```python
from build123d import *


with BuildPart() as part:
    # 스케치2 → 회전1 (revolve)
    with BuildSketch(Plane(origin=(0, 0, 0), x_dir=(0, 0, -1), z_dir=(1, 0, 0))):
        with BuildLine():
            Line((10.1, 0), (12.1, 0))
            ThreePointArc((12.1, 0), (12.521081242, -1.48943877), (11.796548935, -2.857207098))
            ThreePointArc((11.796548935, -2.857207098), (11.081359136, -4.188050052), (11.796542721, -5.518896345))
            ThreePointArc((11.796542721, -5.518896345), (12.753495116, -6.567634704), (13.1, -7.944422413))
            Line((13.1, -7.944422413), (13.1, -19.359260843))
            ThreePointArc((13.1, -19.359260843), (11.975073546, -22.075073546), (9.259260843, -23.2))
            Line((9.259260843, -23.2), (0, -23.2))
            Line((0, -23.2), (0, -20.2))
            Line((0, -20.2), (10.1, -20.2))
            Line((10.1, -20.2), (10.1, 0))
        make_face()
    revolve(axis=Axis((0, -20.2, 0), (0, 1, 0)))


solid = part.part
```
CAD build for the part. Positions are in the model's coordinates, mm. Round coordinates to 2 decimals unless told otherwise and drop trailing zeros. Order: outer loops, then holes, each group sorted by start corner. A loop starts at its lowest first (then second) coordinate and runs counter-clockwise, first axis right, second up. Notation, with made-up numbers: (-1.75, 40.5) -> (19.25, 40.5) arc R21 cw to (19.25, 66.5) -> close; hole circle Ø8 at (49.5, -10.75). An arc over 180 degrees is marked (long way). Write item = value, one per line.
(1) Cut at B-B (z = 0). Write the cut outline in (x, y), plus the area to 3 significant figures.
Answers follow:
outline = (-13.1, -19.36) arc R3.84 ccw to (-9.26, -23.2) -> (9.26, -23.2) arc R3.84 ccw to (13.1, -19.36) -> (13.1, -7.94) arc R2.91 ccw to (11.8, -5.52) arc R1.6 cw to (11.8, -2.86) arc R2.08 ccw to (12.1, 0) -> (10.1, 0) -> (10.1, -20.2) -> (-10.1, -20.2) -> (-10.1, 0) -> (-12.1, 0) arc R2.08 ccw to (-11.8, -2.86) arc R1.6 cw to (-11.8, -5.52) arc R2.91 ccw to (-13.1, -7.94) -> close
area = 178 mm²
(2) Drill centre lines: L1, parallel to Z at x = 0, y = -14.5; L2, parallel to Y at x = 6, z = 6.5. Where is each one in solid material? Low to high.
Answers follow:
L1 = -13.1 to -10.1, 10.1 to 13.1
L2 = -23.2 to -20.2
(3) Cut at D-D (y = -1.5). Write the cut outline in (x, z), plus the area to 3 significant figures.
Answers follow:
outline = circle Ø25.04 at (0, 0); hole circle Ø20.2 at (0, 0)
area = 172 mm²
(4) Flat gauge pins, fed straight in: P1, Ø5, axis at y = -13, z = 6.5, coming from the -X side; P2, Ø4, axis at x = 1, z = 8, coming from the +Y side; P3, Ø2, axis at x = -7, y = -16.5, coming from the -Z side. Where does each tip first touch, or does it go through?
Answers follow:
P1 = -12.47
P2 = -20.2
P3 = -11.65
(5) Pull direction X, two halves, no side cores. Call faces 1 (the flat face through (10, 0, -3)), 2 (the flat face through (0, -20.2, 0)), 3 (the cylindrical face through (-3.034, -9.959, -9.634)), 4 (the cylindrical face through (-12.989, -13.732, 1.705)): +X half, -X half, draft (parallel to the pull), parting line (faces both ways), or undercut.
Answers follow:
face_1 = draft
face_2 = undercut
face_3 = undercut
face_4 = parting line
(6) Cut at C-C (y = -12.25). Write the cut outline in (x, z), plus the area to 3 significant figures.
Answers follow:
outline = circle Ø26.2 at (0, 0); hole circle Ø20.2 at (0, 0)
area = 219 mm²
(7) Cut at A-A (x = 0). Write the cut outline in (y, z), plus the area to 3 significant figures.
Answers follow:
outline = (-23.2, -9.26) arc R3.84 ccw to (-19.36, -13.1) -> (-7.94, -13.1) arc R2.91 ccw to (-5.52, -11.8) arc R1.6 cw to (-2.86, -11.8) arc R2.08 ccw to (0, -12.1) -> (0, -10.1) -> (-20.2, -10.1) -> (-20.2, 10.1) -> (0, 10.1) -> (0, 12.1) arc R2.08 ccw to (-2.86, 11.8) arc R1.6 cw to (-5.52, 11.8) arc R2.91 ccw to (-7.94, 13.1) -> (-19.36, 13.1) arc R3.84 ccw to (-23.2, 9.26) -> close
area = 178 mm²
